Geometry: see drawing. Coordinates: mm, zero at the bounding-box minimum. A direction names the side the tool comes from. Coordinates: 2 decimals unless noted, no trailing zeros. Order: outer loops, then holes, each group sorted by start corner. A loop starts at its lowest first (then second) coordinate and runs counter-clockwise, first axis right, second up. Notation, with made-up numbers: (20, 58) -> (24, 58) arc R14 cw to (24, 62) -> close; hole circle Ø1 at (-33.5, 89.5). An arc over 180 degrees is marked (long way). Write each question's results on one line, items separated by ' | '.
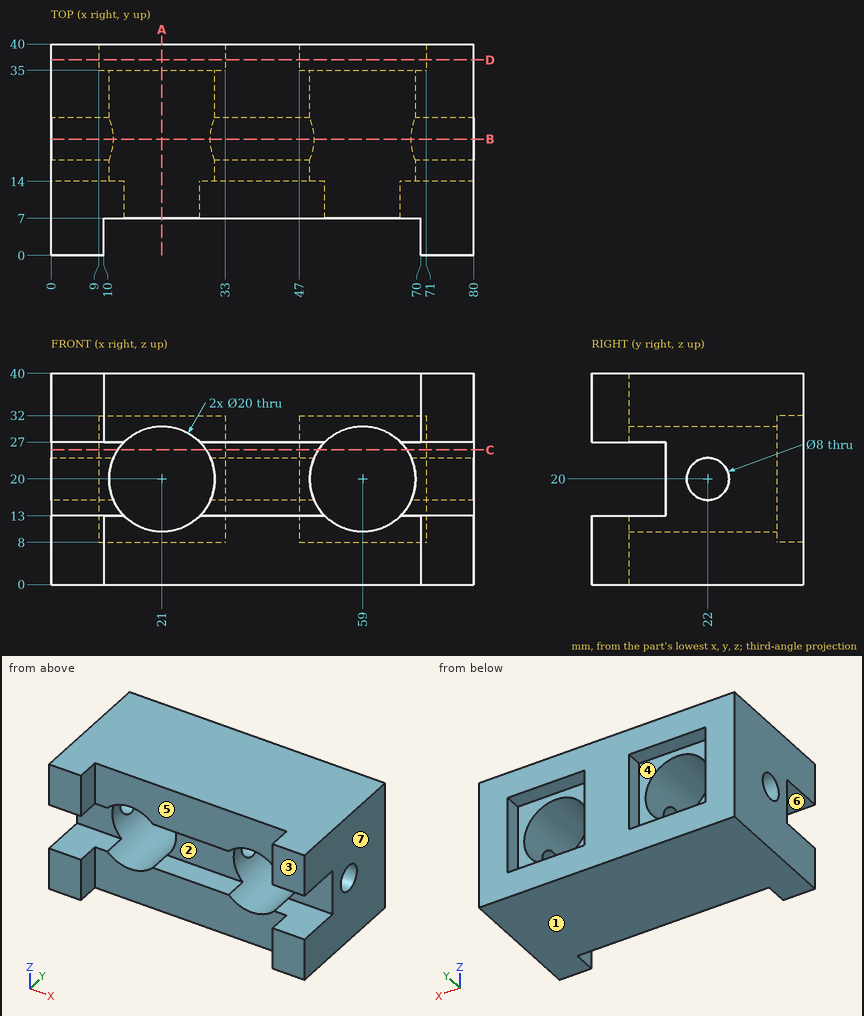
(1) Pin query (flat end, axial travel): P1, Ø15.5, axis at x = 41.5, z = 18, coming from the -Y side; P2, Ø4, axis at x = 71.5, z = 23, coming from the -Y side. Return the tip coordinate at first contact, or that it passes through.
Return value:
P1: y = 7 | P2: y = 14
(2) Cut plane A-A, the plane x = 21. Return loops of the section in (y, z), plus the area to 3 significant figures.
Return value:
outline: (7, 0) -> (40, 0) -> (40, 8) -> (35, 8) -> (35, 10) -> (7, 10) -> close; (7, 30) -> (35, 30) -> (35, 32) -> (40, 32) -> (40, 40) -> (7, 40) -> close | area: 640 mm2
(3) Cut plane D-D, the plane y = 37. Return loops of the section in (x, z), plus the area to 3 significant figures.
Return value:
outline: (0, 0) -> (80, 0) -> (80, 40) -> (0, 40) -> close; hole (9, 8) -> (33, 8) -> (33, 32) -> (9, 32) -> close; hole (47, 8) -> (71, 8) -> (71, 32) -> (47, 32) -> close | area: 2,050 mm2
(4) Cut plane C-C, the plane z = 25.5. Return loops of the section in (x, y), plus the area to 3 significant figures.
Return value:
outline: (0, 14) -> (12.65, 14) -> (12.65, 35) -> (9, 35) -> (9, 40) -> (0, 40) -> close; (29.35, 14) -> (50.65, 14) -> (50.65, 35) -> (47, 35) -> (47, 40) -> (33, 40) -> (33, 35) -> (29.35, 35) -> close; (67.35, 14) -> (80, 14) -> (80, 40) -> (71, 40) -> (71, 35) -> (67.35, 35) -> close | area: 1,140 mm2
(5) Mould query, pull axis Z, two halves, no side actions, for the marked faces 1, 2 and 3. Classes: +Z half, -Z half, draft (parallel to the pull), parting line (faces both ways), or undercut.
Return value:
face 1: -Z half | face 2: undercut | face 3: draft
(6) Line query: line 1 along X through (y, z) = (36, 22); line 2 along Z through (x, y) = (5.5, 22); line 3 along X through (y, z) = (17, 20). Output: solid intervals per line, ascending. Write a range as from..to.
Return value:
line 1: 0..9, 33..47, 71..80 | line 2: 0..16, 24..40 | line 3: 0..11, 31..49, 69..80
(7) Cut plane B-B, the plane y = 22. Return loops of the section in (x, z).
Return value:
outline: (0, 0) -> (80, 0) -> (80, 16) -> (68.17, 16) arc R10 cw to (49.83, 16) -> (30.17, 16) arc R10 cw to (11.83, 16) -> (0, 16) -> close; (0, 24) -> (11.83, 24) arc R10 cw to (30.17, 24) -> (49.83, 24) arc R10 cw to (68.17, 24) -> (80, 24) -> (80, 40) -> (0, 40) -> close
(8) Reachability of the marked faces 4, 5, 6 and 7 from +Z, -Z, +X, -X, +Y, -Y: full face, straight path, thin tool, end or side. Return the list, or none.
Return value:
face 4: +Y | face 5: +Z, -Z, -Y | face 6: +X, -X, -Y | face 7: +Z, -Z, +X, +Y, -Y
